```python
from build123d import *

# Parameters (mm, degrees)
SKETCH3_W           = 120
SKETCH3_H           = 120
BOSS_EXTRUDE2_DEPTH = 50
SKETCH4_R           = 35
BOSS_EXTRUDE3_DEPTH = 25
SKETCH9_R           = 25
CUT_EXTRUDE3_DEPTH  = 186.539753153
FILLET4_R           = 10
FILLET5_R           = 1.5
SHELL2_T            = -2


with BuildPart() as part:
    # Sketch3 → Boss-Extrude2 (new body)
    with BuildSketch(Plane(origin=(0, 0, 0), x_dir=(1, 0, 0), z_dir=(0, 1, 0))):
        with Locations((60, 60)):
            Rectangle(SKETCH3_W, SKETCH3_H)
    extrude(amount=BOSS_EXTRUDE2_DEPTH)

    # Sketch4 → Boss-Extrude3 (add)
    with BuildSketch(Plane(origin=(0, 50, 0), x_dir=(1, 0, 0), z_dir=(0, 1, 0))):
        with Locations(Location((60, 60, 0), (0, 0, 270))):
            Circle(SKETCH4_R)
    extrude(amount=BOSS_EXTRUDE3_DEPTH)

    # Sketch9 → Cut-Extrude3 (cut, through all)
    with BuildSketch(Plane(origin=(0, 75, 0), x_dir=(1, 0, 0), z_dir=(0, 1, 0))):
        with Locations(Location((60, 60, 0), (0, 0, 270))):
            Circle(SKETCH9_R)
    extrude(amount=-CUT_EXTRUDE3_DEPTH, mode=Mode.SUBTRACT)

    # Fillet4
    fillet4_edges = [part.edges().sort_by_distance(p)[0] for p in [
        (60, 50, 0),
        (60, 50, -95),
        (0, 50, -60),
        (60, 50, -120),
        (0, 25, -120),
        (0, 25, 0),
        (120, 25, 0),
        (120, 25, -120),
        (120, 50, -60),
    ]]
    fillet(fillet4_edges, radius=FILLET4_R)

    # Fillet5
    fillet5_edges = [part.edges().sort_by_distance(p)[0] for p in [
        (60, 75, -95),
        (60, 75, -85),
    ]]
    fillet(fillet5_edges, radius=FILLET5_R)

    # Shell2
    shell2_openings = [part.faces().sort_by_distance(p)[0] for p in [
        (60, 0, -1.697056275),
    ]]
    offset(amount=SHELL2_T, openings=shell2_openings, kind=Kind.INTERSECTION)


solid = part.part
```
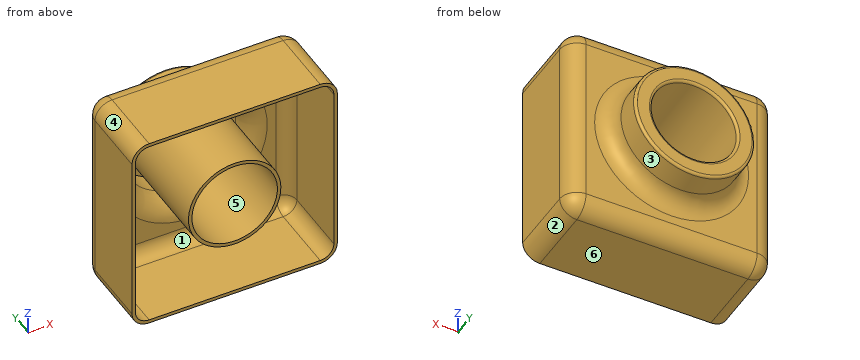
Model file for the job. Use its own axes, mm. Face numbers are marked on the shaded views. A direction names the side the tool comes from. Round coordinates to 2 decimals unless told otherwise and drop trailing zeros. Write each loop counter-clockwise with the first axis right and the second up, starting at its lowest first coordinate (ties: lowest second). Pieces come first, ordered by that corner, then holes. Notation, with made-up numbers: M 63.5,-37.5 L 93.5,-37.5 A11 ccw 93.5,-17.5 Z; hole C 83.5,84 d8. An arc over 180 degrees is marked long. Put each result on its own line as item: value.
Item 1: Tool access for the marked faces 1, 2 and 3: list every direction of +Z, -Z, +X, -X, +Y, -Y with a clear straight run to the whole face (end or side of a thin tool).
Responses:
face 1: -Y
face 2: -Z, +X, +Y, -Y
face 3: +Y
Item 2: Cut at A-A (y = 25). List the corners of the cut face in (x, z), and give its area (3 significant figures).
Responses:
outline: M 0,-110 A10 ccw 10,-120 L 110,-120 A10 ccw 120,-110 L 120,-10 A10 ccw 110,0 L 10,0 A10 ccw 0,-10 Z; C 60,-60 d54; hole M 2,-110 A8 ccw 10,-118 L 110,-118 A8 ccw 118,-110 L 118,-10 A8 ccw 110,-2 L 10,-2 A8 ccw 2,-10 Z; hole C 60,-60 d50
area: 1,240 mm²
Item 3: Mould opens along Z. For the marked faces 4, 5 and 6 say: +Z half, -Z half, draft (parallel to the pull), parting line (faces both ways), or undercut.
Responses:
face 4: +Z half
face 5: undercut
face 6: -Z half
Item 4: Cut at B-B (y = 67). List the corners of the cut face in (x, z), and give its area (3 significant figures).
Responses:
outline: C 60,-60 d70; C 60,-60 d54; hole C 60,-60 d66; hole C 60,-60 d50
area: 754 mm²
Item 5: Flat gauge pins, fed straight in: P1, Ø6, axis at x = 32, y = 49, coming from the +Z side; P2, Ø3, axis at x = 79, z = -103, coming from the -Y side; P3, Ø10, axis at x = 12, z = -101.5, coming from the -Y side. Where does each tip first touch, or does it go through?
Responses:
P1: z = -2
P2: y = 48
P3: y = 47.42
Item 6: Probe L1, parallel to X at y = 64, z = -60; L2, parallel to Z at x = 81, y = 26.5; L3, parallel to X at y = 18.5, z = -31. List the from-to ranges inside material, lowest first. Write a range as from..to.
Responses:
L1: 25..27, 33..35, 85..87, 93..95
L2: -120..-118, -76.97..-73.56, -46.44..-43.03, -2..0
L3: 0..2, 118..120
